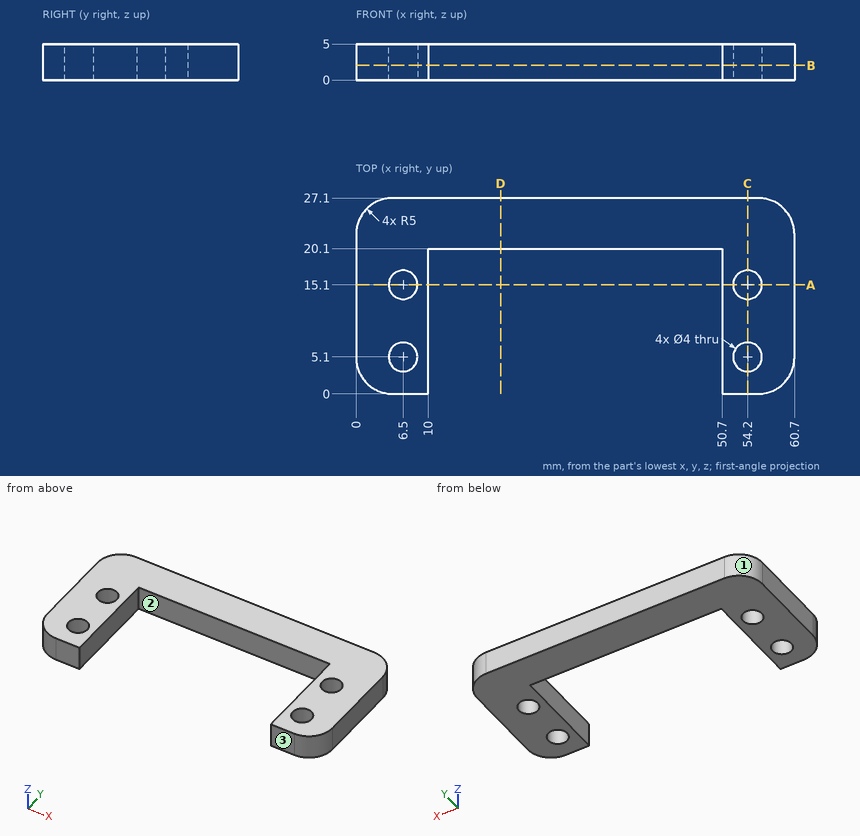
The drawing under review shows one solid part. Ordinate dimensions are in mm from its lowest x, y, z. Round coordinates to 2 decimals unless told otherwise and drop trailing zeros. Write each loop counter-clockwise with the first axis right and the second up, starting at its lowest first coordinate (ties: lowest second). Pieces come first, ordered by that corner, then holes.
(1) We need section D-D on x = 20. Give the boundary of the cut face in (y, z), and give its area (3 significant figures).
(2) Wall thickness on L1, parallel to Y at x = 54.2, z = 3.05; L2, parallel to X at y = 5.75, z = 1.9; L3, parallel to X at y = 13.5, z = 2.85: over which ranges is each line inside the solid? List them lowest first.
(3) We need section A-A on y = 15.1. Give the boundary of the cut face in (x, z), and give its area (3 significant figures).
(4) Mouldability with a two-part tool opening along X and no side actions: class the marked faces 1, 2 and 3 as +X half, -X half, draft (parallel to the pull), parting line (faces both ways), or undercut.
(5) We need section B-B on z = 2.05. Give the boundary of the cut face in (x, y), and give its area (3 significant figures).
(6) We need section C-C on x = 54.2. Give the boundary of the cut face in (y, z).
Findings below:
1. outline: (20.1, 0) - (27.1, 0) - (27.1, 5) - (20.1, 5) - close
1. area: 35.0 mm2
2. L1: y = 0 to 3.1, 7.1 to 13.1, 17.1 to 27.1
2. L2: x = 0 to 4.61, 8.39 to 10, 50.7 to 52.31, 56.09 to 60.7
2. L3: x = 0 to 5.3, 7.7 to 10, 50.7 to 53, 55.4 to 60.7
3. outline: (0, 0) - (4.5, 0) - (4.5, 5) - (0, 5) - close; (8.5, 0) - (10, 0) - (10, 5) - (8.5, 5) - close; (50.7, 0) - (52.2, 0) - (52.2, 5) - (50.7, 5) - close; (56.2, 0) - (60.7, 0) - (60.7, 5) - (56.2, 5) - close
3. area: 60.0 mm2
4. face 1: -X half
4. face 2: undercut
4. face 3: draft
5. outline: (0, 5) arc R5 ccw to (5, 0) - (10, 0) - (10, 20.1) - (50.7, 20.1) - (50.7, 0) - (55.7, 0) arc R5 ccw to (60.7, 5) - (60.7, 22.1) arc R5 ccw to (55.7, 27.1) - (5, 27.1) arc R5 ccw to (0, 22.1) - close; hole circle Ø4 at (6.5, 5.1); hole circle Ø4 at (6.5, 15.1); hole circle Ø4 at (54.2, 5.1); hole circle Ø4 at (54.2, 15.1)
5. area: 755 mm2
6. outline: (0, 0) - (3.1, 0) - (3.1, 5) - (0, 5) - close; (7.1, 0) - (13.1, 0) - (13.1, 5) - (7.1, 5) - close; (17.1, 0) - (27.1, 0) - (27.1, 5) - (17.1, 5) - close
